Source: CAD feature listing. Evaluate the final solid. Frame: model axes, mm. Face numbers are marked on the shaded views. Coordinates: 2 decimals unless noted, no trailing zeros. Loops run counter-clockwise (first coordinate to the right, second up) from the corner with the lowest first, then second, coordinate; pieces in that order, holes last.
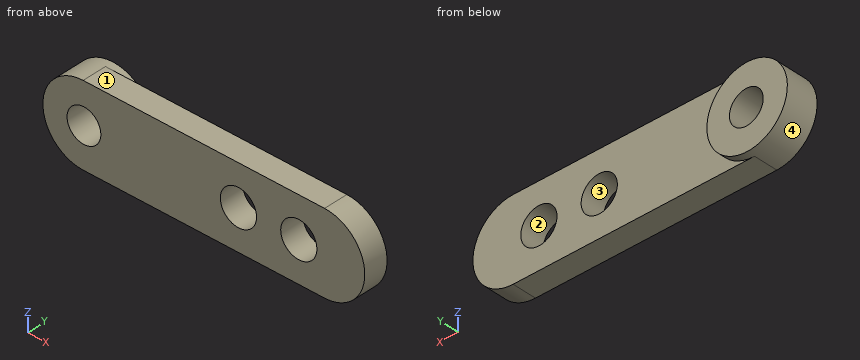
from build123d import *

# Parameters (mm, degrees)
SKETCH1_R           = 2.1
SKETCH1_R_2         = 2.25
BOSS_EXTRUDE1_DEPTH = 3
SKETCH3_R           = 5
SKETCH3_R_2         = 2.1
BOSS_EXTRUDE3_DEPTH = 1


with BuildPart() as part:
    # Sketch1 → Boss-Extrude1 (new body)
    with BuildSketch(Plane(origin=(0, 0, 0), x_dir=(1, 0, 0), z_dir=(0, 1, 0))):
        with BuildLine():
            Line((0, 5), (30, 5))
            ThreePointArc((30, 5), (35, 0), (30, -5))
            Line((30, -5), (0, -5))
            ThreePointArc((0, -5), (-5, 0), (0, 5))
        make_face()
        with Locations(Location((0.1, 0, 0), (0, 0, 270))):
            Circle(SKETCH1_R, mode=Mode.SUBTRACT)
        with Locations(Location((19.3, 0, 0), (0, 0, 270))):
            Circle(SKETCH1_R_2, mode=Mode.SUBTRACT)
        with Locations(Location((26.8, 0, 0), (0, 0, 270))):
            Circle(SKETCH1_R_2, mode=Mode.SUBTRACT)
    extrude(amount=BOSS_EXTRUDE1_DEPTH)

    # Sketch3 → Boss-Extrude3 (add)
    with BuildSketch(Plane(origin=(0, 3, 0), x_dir=(1, 0, 0), z_dir=(0, 1, 0))):
        with Locations(Location((0, 0, 0), (0, 0, 270))):
            Circle(SKETCH3_R)
        with Locations(Location((0.1, 0, 0), (0, 0, 270))):
            Circle(SKETCH3_R_2, mode=Mode.SUBTRACT)
    extrude(amount=BOSS_EXTRUDE3_DEPTH)


solid = part.part
Q1. Section A-A, the plane y = 2.6. Return the cut outline in (x, z), plus the area to 3 significant figures.
Q2. Section B-B, the plane x = 26.8. Return the cut outline in (y, z).
Q3. Draft query along Z for the marked faces 1, 2, 3 and 4. Return one class per face: +Z half, -Z half, draft (parallel to the pull), parting line (faces both ways), or undercut.
Q4. Contact query for flat-ended pins moving along their axis: pin 1 Ø3 at (x, z) = (11.5, -0.5) entering from -Y; pin 2 Ø3.5 at (x, z) = (0.1, 0) entering from +Y; pin 3 Ø3 at (x, z) = (15, -0.5) entering from +Y. Output: stop coordinate, or through.
Q5. Section C-C, the plane z = 0. Return the cut outline in (x, y), plus the area to 3 significant figures.
Q6. Line query: line 1 along X through (y, z) = (2.35, 0); line 2 along Z through (x, y) = (19.5, 1.3); line 3 along Z through (x, y) = (26, 1.9). Output: solid intervals per line, ascending.
Q7. Section D-D, the plane x = 16.5. Return the cut outline in (y, z), plus the area to 3 significant figures.
Derived:
1. outline: (0, -5) - (30, -5) arc R5 ccw to (30, 5) - (0, 5) arc R5 ccw to start; hole circle Ø4.2 at (0.1, 0); hole circle Ø4.5 at (19.3, 0); hole circle Ø4.5 at (26.8, 0)
1. area: 333 mm2
2. outline: (0, -5) - (3, -5) - (3, -2.25) - (0, -2.25) - close; (0, 2.25) - (3, 2.25) - (3, 5) - (0, 5) - close
3. face 1: +Z half
3. face 2: undercut
3. face 3: undercut
3. face 4: parting line
4. pin 1: stops at y = 0
4. pin 2: passes through
4. pin 3: stops at y = 3
5. outline: (-5, 0) - (-2, 0) - (-2, 4) - (-5, 4) - close; (2.2, 0) - (17.05, 0) - (17.05, 3) - (5, 3) - (5, 4) - (2.2, 4) - close; (21.55, 0) - (24.55, 0) - (24.55, 3) - (21.55, 3) - close; (29.05, 0) - (35, 0) - (35, 3) - (29.05, 3) - close
5. area: 86.2 mm2
6. line 1: x = -5 to -2, 2.2 to 17.05, 21.55 to 24.55, 29.05 to 35
6. line 2: z = -5 to -2.24, 2.24 to 5
6. line 3: z = -5 to -2.1, 2.1 to 5
7. outline: (0, -5) - (3, -5) - (3, 5) - (0, 5) - close
7. area: 30.0 mm2
